Can you work these out from the model? Positions are in its coordinate system, mm. Round coordinates to 2 decimals unless told otherwise and drop trailing zeros. Order: outer loops, then holes, each group sorted by start corner. A loop starts at its lowest first (then second) coordinate and runs counter-clockwise, first axis right, second up. Notation, with made-up numbers: (59, 43.5) -> (104, 43.5) arc R25 cw to (104, 68.5) -> close; hole circle Ø7 at (59.25, 75). An arc over 180 degrees is marked (long way). One line per item, written item: value.
Autodesk Inventor part; units mm, degrees
ref_plane "YZ Plane" through (0, 0, 0) normal (1, 0, 0) x (0, 1, 0)
ref_plane "XZ Plane" through (0, 0, 0) normal (0, 1, 0) x (-1, 0, 0)
ref_plane "XY Plane" through (0, 0, 0) normal (0, 0, 1) x (1, 0, 0)
sketch "main" plane through (0, 0, 0) normal (0, 0, 1) x (1, 0, 0)
  circle A0 centre (-14.2783, -9.7185) radius 2.1844
  ellipse E0 centre (34.925, 23.8125) end of major axis (34.925, 33.3375) minor radius 9.5235
  point P0 (-4.2471, 2.7063)
sketch "Sketch1" plane through (0, 0, 0) normal (0, 0, 1) x (1, 0, 0)
  arc A0 (-3.5163, 3.212) -> (-4.7431, -0.4299) centre (0, 0) ccw
  circle A1 centre (0, -25.4) radius 2.0955
  circle A2 centre (-12.7, -25.4) radius 2.0955
  arc A3 (-15.2019, -21.3476) -> (-12.7, -30.1625) centre (-12.7, -25.4) ccw
  line L0 (-12.7, -30.1625) -> (-11.7807, -30.1625)
  arc A4 (-15.2019, -21.3476) -> (-4.7431, -0.4299) centre (-26.8773, -2.4363) ccw
  line L1 (31.75, -25.4) -> (57.15, -25.4) construction
  line L2 (31.75, -25.4) -> (36.5125, -25.4) construction
  circle A5 centre (44.45, -25.4) radius 2.0955
  circle A6 centre (57.15, -25.4) radius 2.0955
  circle A7 centre (69.85, -25.4) radius 5.5499
  arc A8 (63.0478, -32.0675) -> (76.8244, -31.8872) centre (69.85, -25.4) ccw
  circle A9 centre (57.15, -3.403) radius 5.5499
  line L3 (-11.7807, -30.1625) -> (58.513, -30.1625)
  line L4 (81.474, -29.8619) -> (115.2189, -29.8619)
  line L5 (-11.7807, -30.1625) -> (61.6011, -30.1625) construction
  line L6 (78.2653, -29.8619) -> (115.2189, -29.8619) construction
  circle A10 centre (81.2023, 4.7609) radius 5.5499
  arc A11 (83.6265, 13.9723) -> (83.523, 13.9989) centre (81.2023, 4.7609) ccw
  arc A12 (65.1561, 26.0829) -> (83.523, 13.9989) centre (91.6512, 46.3534) ccw
  arc A13 (81.474, -29.8619) -> (76.8244, -31.8872) centre (81.474, -36.2119) ccw
  arc A14 (63.0478, -32.0675) -> (58.513, -30.1625) centre (58.513, -36.5125) ccw
  circle A15 centre (115.2189, -12.3994) radius 11.0998
  arc A16 (132.3184, -15.9417) -> (119.6634, 4.488) centre (115.2189, -12.3994) ccw
  circle A17 centre (104.775, 11.1125) radius 2.0955
  arc A18 (109.4545, 10.2271) -> (100.2659, 12.6454) centre (104.775, 11.1125) ccw
  line L7 (119.6634, 4.488) -> (111.766, 6.5664)
  line L8 (96.4518, 10.5969) -> (83.6265, 13.9723)
  arc A19 (96.4518, 10.5969) -> (100.2659, 12.6454) centre (97.2599, 13.6673) ccw
  arc A20 (109.4545, 10.2271) -> (111.766, 6.5664) centre (112.5741, 9.6369) ccw
  circle A21 centre (130.0641, -33.3375) radius 2.0955
  arc A22 (126.0228, -35.8574) -> (134.3205, -31.2011) centre (130.0641, -33.3375) ccw
  arc A23 (132.3184, -15.9417) -> (134.3205, -31.2011) centre (155.2553, -20.6933) ccw
  arc A24 (126.0228, -35.8574) -> (115.2189, -29.8619) centre (115.2189, -42.5941) ccw
  arc A25 (122.2659, -20.9753) -> (122.2726, -21.4129) centre (155.2553, -20.6933) ccw
  arc A26 (59.7857, -20.6886) -> (58.513, -20.6375) centre (58.513, -36.5125) ccw
  arc A27 (-0.8623, -20.6375) -> (4.8666, -3.0564) centre (-26.8773, -2.4363) ccw
  arc A28 (67.0849, -14.637) -> (58.513, -13.0175) centre (58.513, -36.5125) ccw
  arc A29 (11.0441, -13.0175) -> (12.1111, -7.9042) centre (-26.8773, -2.4363) ccw
  line L9 (4.8666, -3.0564) -> (12.1111, -7.9042)
  line L10 (18.5803, 5.7275) -> (25.1468, 1.3334)
  line L11 (21.4396, 8.2742) -> (27.9161, 3.9403)
  arc A30 (15.3458, -20.6375) -> (17.8676, -13.0175) centre (-26.8773, -2.4363) ccw
  line L12 (17.8676, -13.0175) -> (11.0441, -13.0175)
  line L13 (15.3458, -20.6375) -> (-0.8623, -20.6375)
  line L14 (38.7856, -20.6375) -> (38.7856, -13.0175)
  line L15 (41.1925, -20.6375) -> (41.1925, -13.0175)
  line L16 (44.2415, -13.0175) -> (44.2415, -20.6375)
  line L17 (58.513, -13.0175) -> (44.2415, -13.0175)
  line L18 (41.1925, -13.0175) -> (38.7856, -13.0175)
  line L19 (58.513, -20.6375) -> (44.2415, -20.6375)
  line L20 (41.1925, -20.6375) -> (38.7856, -20.6375)
  arc A31 (41.2533, 43.0681) -> (41.1925, 43.0108) centre (44.4887, 39.5733) ccw
  line L21 (15.3458, 3.189) -> (22.0356, -1.2876)
  arc A32 (15.3458, 3.189) -> (18.5803, 5.7275) centre (-22.4149, 54.6332) ccw
  arc A33 (21.4396, 8.2742) -> (29.3428, 17.3034) centre (-22.4149, 54.6332) ccw
  arc A34 (22.0356, -1.2876) -> (25.1468, 1.3334) centre (-22.4149, 54.6332) ccw
  arc A35 (40.5702, 20.9307) -> (41.1925, 20.8107) centre (44.4887, 39.5733) ccw
  arc A36 (27.9161, 3.9403) -> (36.2836, 13.9213) centre (-22.4149, 54.6332) ccw
  arc A37 (83.6265, 13.9723) -> (83.523, 13.9989) centre (81.2023, 4.7609) ccw
  arc A38 (112.1958, -29.8619) -> (117.1762, -30.0133) centre (115.2189, -12.3994) ccw
  arc A39 (67.0849, -14.637) -> (59.7857, -20.6886) centre (69.85, -25.4) ccw
  arc A40 (59.8098, -30.1625) -> (59.882, -30.3118) centre (69.85, -25.4) ccw
  arc A41 (79.9432, -30.0492) -> (80.0274, -29.8619) centre (69.85, -25.4) ccw
  arc A42 (81.474, -14.2875) -> (76.801, -14.7913) centre (81.474, -36.2119) ccw
  arc A43 (80.6713, -18.7848) -> (76.801, -14.7913) centre (69.85, -25.4) ccw
  arc A44 (81.474, -18.7664) -> (80.6713, -18.7848) centre (81.474, -36.2119) ccw
  line L22 (81.474, -18.7664) -> (97.0069, -18.7664)
  arc A45 (96.0187, -14.2875) -> (97.0069, -18.7664) centre (115.2189, -12.3994) ccw
  line L23 (96.0187, -14.2875) -> (81.474, -14.2875)
  circle A46 centre (62.7575, 21.436) radius 2.0955
  arc A47 (10.6679, 3.212) -> (25.8705, 23.0519) centre (-26.8733, 47.7228) ccw
  arc A48 (30.8454, 24.0889) -> (60.215, 26.2096) centre (44.4887, 39.5733) ccw
  arc A49 (29.3428, 17.3034) -> (36.2836, 13.9213) centre (44.4887, 39.5733) ccw
  arc A50 (30.8454, 24.0889) -> (25.8705, 23.0519) centre (28.7464, 21.7067) ccw
  arc A51 (65.1561, 26.0829) -> (60.215, 26.2096) centre (62.6345, 24.1537) ccw
  circle A52 centre (0, 0) radius 2.0955
  line L24 (-3.5163, 3.212) -> (10.6679, 3.212)
  point P0 (-1.8077, 4.4061)
  point P1 (107.9569, 7.5689)
  point P2 (100.2609, 9.5944)
  point P3 (9.126, 4.4208)
  point P4 (41.1925, 20.8107)
  dimension "d7" = 22.225
  dimension "d25" = 4.191
  dimension "d26" = 4.191
  dimension "d30" = 11.0998
  dimension "d31" = 11.0998
  dimension "d38" = 6.35
  dimension "d43" = 4.191
  dimension "d44" = 9.525
  dimension "d47" = 9.525
  dimension "d54" = 4.191
  dimension "d56" = 12.7
  dimension "d58" = 41.275
  dimension "d60" = 3.175
extrude "Extrusion1" add sketch "Sketch1" along normal blind 1.5875 contours L24 A47 A50 A48 A51 A12 A11 L8 A19 A18 A20 L7 A16 A23 A22 A24 L4 A13 A8 A14 L3 L0 A3 A4 A0
properties part number "reservoir_mount_inner" material "Acetal Resin, White"
Q1. I want a section at B-B on x = 121.5. List the corners of the cut face in (y, z) for me, plus the area to 3 significant figures.
Answers below:
outline: (-31.52, 0) -> (-21.55, 0) -> (-21.55, 1.59) -> (-31.52, 1.59) -> close; (-3.25, 0) -> (3.89, 0) -> (3.89, 1.59) -> (-3.25, 1.59) -> close
area: 27.2 mm^2
Q2. Will these pins go through, and if not, where does the flat tip stop? pin 1 Ø3.5 at (x, y) = (104.78, 11.11) entering from +Z; pin 2 Ø0.5 at (x, z) = (90, 0.5) entering from -Y.
Answers below:
pin 1: through
pin 2: y = -29.86
Q3. I want a section at C-C on z = 0.75. Give the number of separate pieces and of enclosed holes in the cut face, plus the area to 3 significant figures.
Answers below:
separate pieces: 1
enclosed holes: 18
area: 4,930 mm^2
Q4. I want a section at A-A on x = 48. List the corners of the cut face in (y, z) for me, plus the area to 3 significant figures.
Answers below:
outline: (-30.16, 0) -> (-20.64, 0) -> (-20.64, 1.59) -> (-30.16, 1.59) -> close; (-13.02, 0) -> (19.24, 0) -> (19.24, 1.59) -> (-13.02, 1.59) -> close
area: 66.3 mm^2
Q5. We'd pull the mould along X, two halves only. Please class faces 1 (the face through (46.204, 19.007, 0.783)), 2 (the face through (90.13, 12.26, 0.78)), 3 (the face through (19.453, 12.447, 0.783)), 4 (the face through (58, -12, 1.588)): released by +X, released by -X, zero draft, split by the parting line, or undercut.
Answers below:
face 1: undercut
face 2: undercut
face 3: released by -X
face 4: zero draft
Q6. Please list where these lines run through material, in increasing order: line 1 along Y through (x, z) = (57.15, 0.5); line 2 along X through (y, z) = (-33.5, 1.05); line 3 along X through (y, z) = (1.5, 0.15).
Answers below:
line 1: -30.16 to -27.5, -23.3 to -20.64, -13.02 to -8.95, 2.15 to 23.28
line 2: 64.84 to 74.86, 124.13 to 127.97, 132.15 to 134.82
line 3: -4.52 to -1.46, 1.46 to 17.87, 24.9 to 54.55, 59.75 to 76.71, 85.69 to 125.79
